Could you check a few things on this model? Use its own coordinates, in mm. Give positions to 0.01 mm unless a question says otherwise; leave off trailing zeros. Write each loop counter-clockwise with the first axis right and the second up, starting at its lowest first coordinate (ties: lowest second). Pieces come first, ordered by that corner, then holes. Notation, with made-up numbers: M 62.25,-34 L 118.25,-34 A16 ccw 118.25,-22 Z; hole C -30.75,-34 d6. An arc over 180 degrees is marked long. One line per item, written item: value.
```python
from build123d import *

# Parameters (mm, degrees)
SKETCH1_W           = 82.5
SKETCH1_H           = 57.8
BOSS_EXTRUDE1_DEPTH = 4.8
SKETCH2_R           = 12.5
CUT_EXTRUDE1_DEPTH  = 4.8
CUT_EXTRUDE2_DEPTH  = 2.8


with BuildPart() as part:
    # Sketch1 → Boss-Extrude1 (new body)
    with BuildSketch(Plane(origin=(0, 0, 0), x_dir=(1, 0, 0), z_dir=(0, 1, 0))):
        with Locations((20.883891213, 18.735983264)):
            Rectangle(SKETCH1_W, SKETCH1_H)
    extrude(amount=BOSS_EXTRUDE1_DEPTH)

    # Sketch2 → Cut-Extrude1 (cut)
    with BuildSketch(Plane(origin=(0, 4.8, 0), x_dir=(1, 0, 0), z_dir=(0, 1, 0))):
        with Locations((35.633891213, 22.835983264)):
            Circle(SKETCH2_R)
        Polygon((41.133891213, -10.164016736), (62.133891213, 24.835983264), (62.133891213, -10.164016736), align=None)
    extrude(amount=-CUT_EXTRUDE1_DEPTH, mode=Mode.SUBTRACT)

    # Sketch3 → Cut-Extrude2 (cut)
    with BuildSketch(Plane(origin=(0, 4.8, 0), x_dir=(1, 0, 0), z_dir=(0, 1, 0))):
        with BuildLine():
            ThreePointArc((30.533891213, 34.248257358), (33.026538742, 35.061027766), (35.633891213, 35.335983264))
            Line((35.633891213, 35.335983264), (35.633891213, 37.535983264))
            ThreePointArc((35.633891213, 37.535983264), (33.04334785, 37.30592055), (30.533891213, 36.622933615))
            Line((30.533891213, 36.622933615), (30.533891213, 34.248257358))
        make_face()
        with BuildLine():
            Line((35.633891213, 37.535983264), (35.633891213, 35.335983264))
            ThreePointArc((35.633891213, 35.335983264), (38.241243685, 35.061027766), (40.733891213, 34.248257358))
            Line((40.733891213, 34.248257358), (40.733891213, 36.622933615))
            ThreePointArc((40.733891213, 36.622933615), (38.224434576, 37.30592055), (35.633891213, 37.535983264))
        make_face()
        with BuildLine():
            ThreePointArc((48.067210494, 21.546575776), (47.524766551, 18.981494489), (46.459208761, 16.585983264))
            Line((46.459208761, 16.585983264), (48.364464649, 15.485983264))
            ThreePointArc((48.364464649, 15.485983264), (49.460496176, 17.844490982), (50.123740459, 20.359237647))
            Line((50.123740459, 20.359237647), (48.067210494, 21.546575776))
        make_face()
        with BuildLine():
            Line((48.364464649, 15.485983264), (46.459208761, 16.585983264))
            ThreePointArc((46.459208761, 16.585983264), (44.917414079, 14.465427535), (42.967210494, 12.713116657))
            Line((42.967210494, 12.713116657), (45.023740459, 11.525778528))
            ThreePointArc((45.023740459, 11.525778528), (46.869952814, 13.357538258), (48.364464649, 15.485983264))
        make_face()
        with BuildLine():
            Line((22.903317778, 15.485983264), (24.808573666, 16.585983264))
            ThreePointArc((24.808573666, 16.585983264), (23.743015876, 18.981494489), (23.200571933, 21.546575776))
            Line((23.200571933, 21.546575776), (21.144041968, 20.359237647))
            ThreePointArc((21.144041968, 20.359237647), (21.80728625, 17.844490982), (22.903317778, 15.485983264))
        make_face()
        with BuildLine():
            ThreePointArc((28.300571933, 12.713116657), (26.350368348, 14.465427535), (24.808573666, 16.585983264))
            Line((24.808573666, 16.585983264), (22.903317778, 15.485983264))
            ThreePointArc((22.903317778, 15.485983264), (24.397829613, 13.357538258), (26.244041968, 11.525778528))
            Line((26.244041968, 11.525778528), (28.300571933, 12.713116657))
        make_face()
    extrude(amount=-CUT_EXTRUDE2_DEPTH, mode=Mode.SUBTRACT)


solid = part.part
```
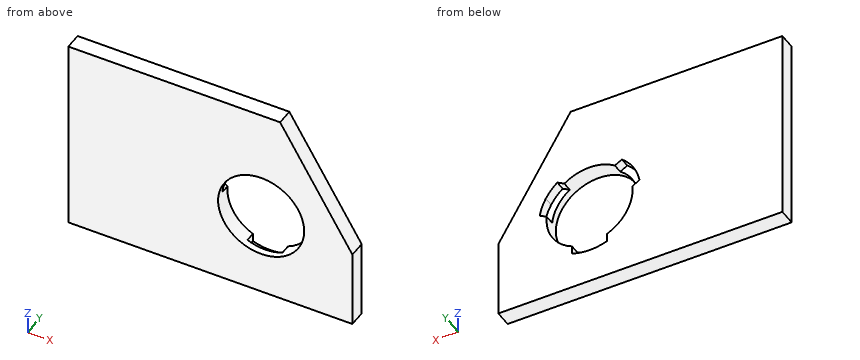
1) If we section it at D-D, the plane z = -18: Write out the boundary of the cut face in (x, y), then the cut area to 3 significant figures.
Outcome:
outline: M -20.37,0 L 24.11,0 L 24.11,2 L 21.75,2 L 21.75,4.8 L -20.37,4.8 Z; M 47.16,0 L 58.03,0 L 58.03,4.8 L 49.52,4.8 L 49.52,2 L 47.16,2 Z
area: 252 mm^2
2) If we section it at B-B, the plane y = 2.8: Write out the boundary of the cut face in (x, z).
Outcome:
outline: M -20.37,-47.64 L 62.13,-47.64 L 62.13,-24.84 L 41.13,10.16 L -20.37,10.16 Z; hole M 21.14,-20.36 L 23.2,-21.55 A12.5 ccw 30.53,-34.25 L 30.53,-36.62 A14.7 ccw 40.73,-36.62 L 40.73,-34.25 A12.5 ccw 48.07,-21.55 L 50.12,-20.36 A14.7 ccw 45.02,-11.53 L 42.97,-12.71 A12.5 ccw 28.3,-12.71 L 26.24,-11.53 A14.7 ccw Z
3) Please list where these lines run through material, in increasing order: L1, parallel to Z at x = 31, y = 1.9; L2, parallel to Z at x = 27.5, y = 1.9; L3, parallel to X at y = 0.9, z = -9. Write a range as from..to.
Outcome:
L1: z = -47.64..-34.45, -11.23..10.16
L2: z = -47.64..-32.33, -13.34..10.16
L3: x = -20.37..52.63
4) If we section it at A-A, the plane x = 39: Write out the boundary of the cut face in (y, z), then the cut area to 3 significant figures.
Outcome:
outline: M 0,-47.64 L 4.8,-47.64 L 4.8,-37.15 L 2,-37.15 L 2,-34.87 L 0,-34.87 Z; M 0,-10.8 L 4.8,-10.8 L 4.8,10.16 L 0,10.16 Z
area: 156 mm^2
5) If we section it at C-C, the plane z = -31.5: Write out the boundary of the cut face in (x, y), then the cut area to 3 significant figures.
Outcome:
outline: M -20.37,0 L 26.62,0 L 26.62,4.8 L -20.37,4.8 Z; M 44.64,0 L 62.13,0 L 62.13,4.8 L 44.64,4.8 Z
area: 310 mm^2
6) I'm going to push flat-ended pins straight in: pin 1 (2 mm diameter, centred on x = 26, z = -15.5, fed in from +Y); pin 2 (5.5 mm diameter, centred on x = 48, z = -17, fed in from +Y). Where does each tip first touch, or does it pass through?
Outcome:
pin 1: stops at y = 2
pin 2: stops at y = 4.8
